```python
from build123d import *

# Parameters (mm, degrees)
SKETCH1_W               = 20
SKETCH1_H               = 20
BOSS_EXTRUDE1_DEPTH     = 3
CUT_EXTRUDE1_DEPTH      = 1
CUT_EXTRUDE1_DEPTH_BACK = 4
CUT_EXTRUDE2_START      = -4
SKETCH3_W               = 5
SKETCH3_H               = 3
CUT_EXTRUDE2_DEPTH      = 5


with BuildPart() as part:
    # Sketch1 → Boss-Extrude1 (new body)
    with BuildSketch(Plane(origin=(0, 0, 0), x_dir=(1, 0, 0), z_dir=(0, 1, 0))):
        Rectangle(SKETCH1_W, SKETCH1_H)
    extrude(amount=BOSS_EXTRUDE1_DEPTH)

    # Sketch2 → Cut-Extrude1 (cut, two sides)
    with BuildSketch(Plane(origin=(0, 3, 0), x_dir=(1, 0, 0), z_dir=(0, 1, 0))) as cut_extrude1_sk:
        Polygon((-5, -10), (-10, -5), (-10, -10), align=None)
        Polygon((0, -5), (-5, -10), (5, -10), align=None)
        Polygon((10, -5), (5, -10), (10, -10), align=None)
    extrude(amount=CUT_EXTRUDE1_DEPTH, mode=Mode.SUBTRACT)
    extrude(cut_extrude1_sk.sketch, amount=-CUT_EXTRUDE1_DEPTH_BACK, mode=Mode.SUBTRACT)

    # Sketch3 → Cut-Extrude2 (cut)
    with BuildSketch(Plane(origin=(0, 3, 0), x_dir=(1, 0, 0), z_dir=(0, 1, 0)).offset(CUT_EXTRUDE2_START)):
        with Locations((-5, 8.5)):
            Rectangle(SKETCH3_W, SKETCH3_H)
    cut_extrude2 = extrude(amount=CUT_EXTRUDE2_DEPTH, mode=Mode.SUBTRACT)

    # Mirror1: Cut-Extrude2 across plane
    add(cut_extrude2.mirror(Plane(origin=(0, 0, 0), x_dir=(0, 0, 1), z_dir=(1, 0, 0))), mode=Mode.SUBTRACT)


solid = part.part
```
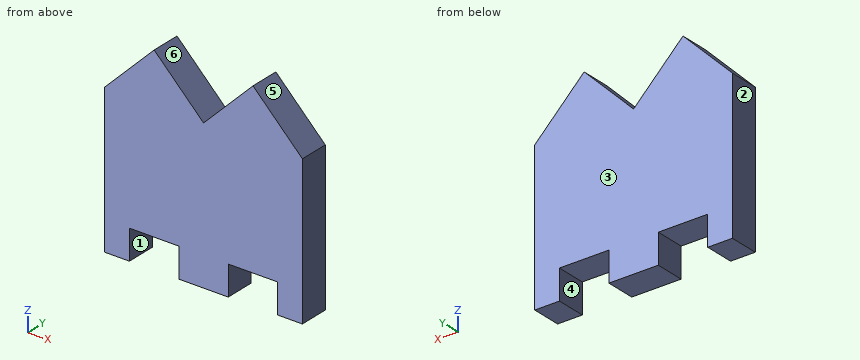
The model under review builds one solid part; all positions refer to its coordinate system, in mm. Face numbers are marked on the shaded views. A direction names the side the tool comes from. Round coordinates to 2 decimals unless told otherwise and drop trailing zeros. Loops run counter-clockwise (first coordinate to the right, second up) from the corner with the lowest first, then second, coordinate; pieces in that order, holes last.
Item 1: Take a section at C-C (z = 6.5). Write out the cut boundary in (x, y), then the cut area to 3 significant figures.
Determined:
outline: (-8.5, 0) - (-1.5, 0) - (-1.5, 3) - (-8.5, 3) - close; (1.5, 0) - (8.5, 0) - (8.5, 3) - (1.5, 3) - close
area: 42.0 mm2
Item 2: Take a section at B-B (y = 1.45). Write out the cut boundary in (x, z).
Determined:
outline: (-10, -10) - (-7.5, -10) - (-7.5, -7) - (-2.5, -7) - (-2.5, -10) - (2.5, -10) - (2.5, -7) - (7.5, -7) - (7.5, -10) - (10, -10) - (10, 5) - (5, 10) - (0, 5) - (-5, 10) - (-10, 5) - close
Item 3: Take a section at A-A (z = -7.75). Write out the cut boundary in (x, y), then the cut area to 3 significant figures.
Determined:
outline: (-10, 0) - (-7.5, 0) - (-7.5, 3) - (-10, 3) - close; (-2.5, 0) - (2.5, 0) - (2.5, 3) - (-2.5, 3) - close; (7.5, 0) - (10, 0) - (10, 3) - (7.5, 3) - close
area: 30.0 mm2
Item 4: For the marked faces 4, 5 and 6, list the 3-axis set-ups (+Z, -Z, +X, -X, +Y, -Y) from which the entire face can be reached by the end or side of a thin tool; tool diameter is ignored.
Determined:
face 4: -Z, +Y, -Y
face 5: +Z, +X, +Y, -Y
face 6: +Z, +Y, -Y
Item 5: Clearance check with a flat-ended pin moving along its axis: pin 1 Ø0.9 at (x, y) = (5.5, 1) entering from -Z. State where the tip first meets the part, or that it passes through.
Determined:
pin 1: stops at z = -7
Item 6: Take a section at D-D (x = -3.5). Write out the cut boundary in (y, z), then the cut area to 3 significant figures.
Determined:
outline: (0, -7) - (3, -7) - (3, 8.5) - (0, 8.5) - close
area: 46.5 mm2
Item 7: Mouldability with a two-part tool opening along X and no side actions: class the marked faces 1, 2 and 3 as released by +X, released by -X, zero draft, split by the parting line, or undercut.
Determined:
face 1: undercut
face 2: released by -X
face 3: zero draft
Item 8: For line 1 (X direction, y = 1, z = -8); line 2 (X direction, y = 0.65, z = 6.5); line 3 (Z direction, x = 1, y = 2.65), list the stretches that pass through material, from the lowest coordinate up.
Determined:
line 1: x = -10 to -7.5, -2.5 to 2.5, 7.5 to 10
line 2: x = -8.5 to -1.5, 1.5 to 8.5
line 3: z = -10 to 6
